Build history of the part. All positions in model axes, mm. Round coordinates to 2 decimals unless told otherwise and drop trailing zeros. Write each loop counter-clockwise with the first axis right and the second up, starting at its lowest first coordinate (ties: lowest second). Pieces come first, ordered by that corner, then holes. Notation, with made-up numbers: M 64.25,81.25 L 94.25,81.25 A22 cw 94.25,115.25 Z; hole C 39.5,-2 d6. An arc over 180 degrees is marked long. Write item = value, one per line. Start each with the question number.
Q1. Drop flat-ended pins along their axis: P1, Ø3, axis at y = 2, z = 45.5, coming from the +X side; P2, Ø4, axis at y = 1.5, z = 45.5, coming from the +X side; P3, Ø2, axis at y = -2, z = 57.5, coming from the -X side; P4, Ø3, axis at x = 2.5, z = 67, coming from the +Y side. Give the stop position or say it passes through.
Q2. Band-saw the part on A-A on z = 32.5. Write the cut outline in (x, y) (1 decimal), plus the area to 3 significant figures.
Q3. Pull direction Y, two halves, no side cores. Call faces 1 (the cylindrical face through (-3.78, 2.9, 63.14)), 2 (the flat face through (2, 0, 0)), 3 (the cylindrical face through (0.632, 1.525, 6.233)): released by +Y, released by -Y, zero draft, split by the parting line, or undercut.
Autodesk Inventor part; units mm, degrees
ref_plane "YZ Plane" through (0, 0, 0) normal (1, 0, 0) x (0, 1, 0)
ref_plane "XZ Plane" through (0, 0, 0) normal (0, 1, 0) x (-1, 0, 0)
ref_plane "XY Plane" through (0, 0, 0) normal (0, 0, 1) x (1, 0, 0)
sketch "Sketch1" plane through (0, 0, 0) normal (0, 0, 1) x (1, 0, 0)
  circle A0 centre (0, 0) radius 4.7625
  dimension "d0" = 9.525
extrude "Extrusion1" add sketch "Sketch1" along normal blind 128.5875
sketch "Sketch2" plane through (0, 0, 0) normal (0, 0, -1) x (-1, 0, 0)
  point P0 (0, 0)
  point P1 (0, 0)
hole "Hole1" at (0, 0, 0) direction (0, 0, 1) diameter 3.302 depth 12.2936 tip angle 118
chamfer "Chamfer1" distance 0.508 angle 45 1 edges at (-4.7625, 0, 128.5875)
properties part number "post"
Conclusion:
q1.P1 = 4.74
q1.P2 = 4.76
q1.P3 = -4.66
q1.P4 = 4.66
q2.outline = C 0,0 d9.5
q2.area = 71.3 mm^2
q3.face_1 = split by the parting line
q3.face_2 = zero draft
q3.face_3 = undercut
